Study the drawing (mm; zero at the part's minimum x, y, z) and answer. Give positions to 0.01 mm unless a question says otherwise; leave off trailing zeros. Loops run counter-clockwise (first coordinate to the right, second up) from the corner with the lowest first, then second, coordinate; pieces in that order, holes last. Notation, with made-up numbers: (74.25, -36.75) -> (128.25, -36.75) arc R3 cw to (128.25, -32.75) -> close; hole circle Ø11 at (49.5, 17.5). An arc over 180 degrees is marked (long way). One line per question, with ' | ' between items. Start each with the question number.
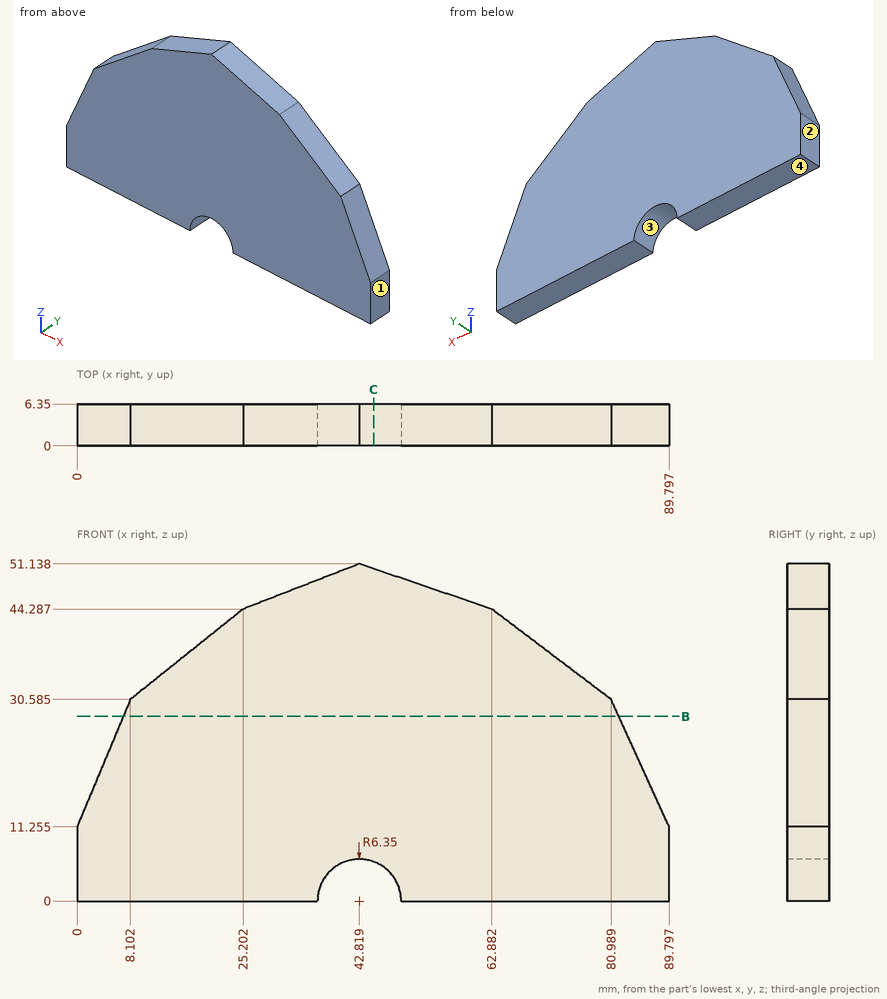
1. The part is cut by section B-B (z = 28). Write down the section's boundary in (x, y).
2. This flat-tipped pin is pushed along its axis until it touches: pin 1 Ø1 at (y, z) = (5, 41.5) entering from +X (1 decimal). Where does it stop, or does it pass through?
3. Straight lines are drawn through the part: L1, parallel to X at y = 1.25, z = 2 (1 decimal); L2, parallel to Z at x = 77, y = 4.5 (1 decimal); L3, parallel to Z at x = 17, y = 3.25 (1 decimal). For each, find the intervals that lie inside material, in ascending order.
4. The part is cut by section C-C (x = 45). Write down the section's boundary in (y, z), plus the area to 3 significant figures.
5. Determine the mould class of the marked faces 1, 2, 3 and 4 for opening direction X: released by +X, released by -X, zero draft, split by the parting line, or undercut.
Check sheet entries:
1) outline: (7.02, 0) -> (82.17, 0) -> (82.17, 6.35) -> (7.02, 6.35) -> close
2) pin 1: stops at x = 67.2
3) L1: x = 0 to 36.8, 48.8 to 89.8 | L2: z = 0 to 33.6 | L3: z = 0 to 37.7
4) outline: (0, 5.96) -> (6.35, 5.96) -> (6.35, 50.39) -> (0, 50.39) -> close | area: 282 mm^2
5) face 1: released by +X | face 2: released by -X | face 3: undercut | face 4: zero draft
